from build123d import *

# Parameters (mm, degrees)
F1_DEPTH = 16
F2_T     = -1.5
F4_DEPTH = 100
F6_DEPTH = 25
F7_R     = 2


with BuildPart() as f1:
    # F0 (on Front) → F1 (new body)
    with BuildSketch(Plane.XZ):
        Polygon((32.5, -9), (32.5, 9), (-32.5, 9), (-32.5, -9), (-6, -9), (-6, -32), (6, -32), (6, -9), align=None)
    extrude(amount=F1_DEPTH)

    # F2
    f2_openings = [f1.faces().sort_by_distance(p)[0] for p in [
        (0, -16, -3.912863),
    ]]
    offset(amount=F2_T, openings=f2_openings, kind=Kind.INTERSECTION)

    # F3 (on face) → F4 (cut)
    with BuildSketch(Plane.YZ.offset(32.5)):
        with BuildLine():
            ThreePointArc((-7.5, -5), (-3.9644660941, -3.5355339059), (-2.5, 0))
            ThreePointArc((-2.5, 0), (-3.9336885694, 3.5044860935), (-7.4125691119, 4.9992355255))
            Line((-7.4125691119, 4.9992355255), (-7.5874308881, 4.9992355255))
            ThreePointArc((-7.5874308881, 4.9992355255), (-12.4994020552, 0.0773245797), (-7.7419960904, -4.9941403557))
            Line((-7.7419960904, -4.9941403557), (-7.5, -5))
        make_face()
        with BuildLine():
            Line((-7.5874308881, 4.9992355255), (-7.4125691119, 4.9992355255))
            ThreePointArc((-7.4125691119, 4.9992355255), (-7.5, 5), (-7.5874308881, 4.9992355255))
        make_face()
        with BuildLine():
            ThreePointArc((-7.7419960904, -4.9941403557), (-7.6210335111, -4.9985348743), (-7.5, -5))
            Line((-7.5, -5), (-7.7419960904, -4.9941403557))
        make_face()
        with BuildLine():
            ThreePointArc((-7.7419960904, -4.9941403557), (-12.4994020552, 0.0773245797), (-7.5874308881, 4.9992355255))
            Line((-7.5874308881, 4.9992355255), (-16, 4.9992355255))
            Line((-16, 4.9992355255), (-16, -4.7941827215))
            Line((-16, -4.7941827215), (-7.7419960904, -4.9941403557))
        make_face()
    extrude(amount=-F4_DEPTH, mode=Mode.SUBTRACT)

    # F5 (on face) → F6 (cut)
    with BuildSketch(Plane(origin=(0, 0, -32), x_dir=(1, 0, 0), z_dir=(0, 0, -1))):
        with BuildLine():
            ThreePointArc((-3.5, 6), (0, 2.5), (3.5, 6))
            ThreePointArc((3.5, 6), (0, 9.5), (-3.5, 6))
        make_face()
        with BuildLine():
            ThreePointArc((-3.5, 6), (0, 9.5), (3.5, 6))
            Line((3.5, 6), (3.5, 16))
            Line((3.5, 16), (-3.5, 16))
            Line((-3.5, 16), (-3.5, 6))
        make_face()
    extrude(amount=-F6_DEPTH, mode=Mode.SUBTRACT)

    # F7
    f7_edges = [f1.edges().sort_by_distance(p)[0] for p in [
        (-32.5, -8, -9),
        (-6, -8, -9),
        (-6, -8, -32),
        (6, -8, -32),
        (6, -8, -9),
        (32.5, -8, -9),
        (32.5, -8, 9),
        (-32.5, -8, 9),
    ]]
    fillet(f7_edges, radius=F7_R)


solid = f1.part
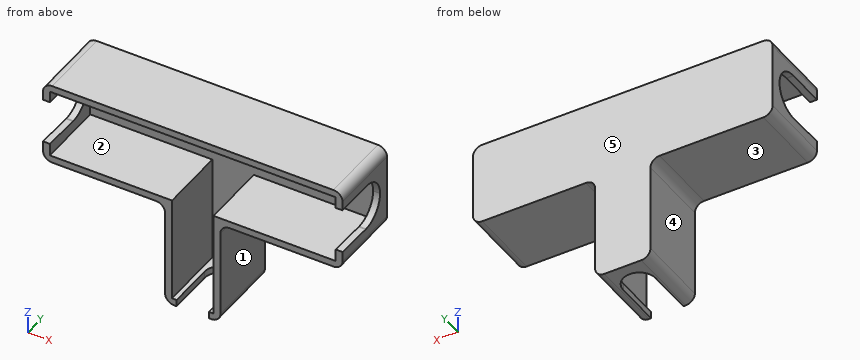
Read the model definition and answer for the solid it produces. Units are mm, in the model's axes. Face numbers are marked on the shaded views. A direction names the side the tool comes from. Round coordinates to 2 decimals unless told otherwise and drop trailing zeros. Order: outer loops, then holes, each group sorted by start corner. A loop starts at its lowest first (then second) coordinate and runs counter-clockwise, first axis right, second up.
1) Flat-ended cylindrical pins translate along their axes: pin 1 (7 mm diameter, centred on y = -6.5, z = -1.5, fed in from +X); pin 2 (1.2 mm diameter, centred on x = -32, y = -11.5, fed in from -Z); pin 3 (6 mm diameter, centred on x = -17, y = -7, fed in from -Z); pin 4 (8 mm diameter, centred on y = -8.5, z = -16.5, fed in from -X). Find the tip coordinate at first contact, or state that the pin passes through.
2) The mould has two halves that part along Y. Classify the marked faces 4 and 5: released by +Y, released by -Y, zero draft, split by the parting line, or undercut.
3) The part is cut by section A-A on x = -25.5. Write down the section's boundary in (y, z).
4) The part is cut by section B-B on z = -17.5. Write down the section's boundary in (x, y), plus the area to 3 significant figures.
5) Straight lines are drawn through the part: L1, parallel to Z at x = -16, y = -2.25; L2, parallel to X at y = -9.25, z = 7; L3, parallel to X at y = -4, z = -16.5. For each, find the intervals that lie inside material, in ascending order.
6) For the marked faces 1, 2 and 3, determine the directions among +Z, -Z, +X, -X, +Y, -Y from which every point of the face is accessible in a straight line to the end or side of a thin tool.
7) The part is cut by section C-C on y = -12.75. Give the number of separate pieces and of enclosed holes in the cut face, plus the area to 3 significant figures.
Resolved:
1. pin 1: stops at x = 32.5
1. pin 2: stops at z = -8.79
1. pin 3: stops at z = -9
1. pin 4: stops at x = -6
2. face 4: zero draft
2. face 5: released by +Y
3. outline: (-16, -9) - (0, -9) - (0, 9) - (-16, 9) - (-16, 7.5) - (-1.5, 7.5) - (-1.5, -7.5) - (-16, -7.5) - close
4. outline: (-6, -16) - (-4.5, -16) - (-4.5, -1.5) - (4.5, -1.5) - (4.5, -16) - (6, -16) - (6, 0) - (-6, 0) - close
4. area: 61.5 mm2
5. L1: z = -9 to -7.5, 7.5 to 9
5. L2: x = -32.5 to -31, 31 to 32.5
5. L3: x = -6 to -4.5, 4.5 to 6
6. face 1: -Z, +X, +Y, -Y
6. face 2: -Y
6. face 3: -Z, -X, +Y, -Y
7. separate pieces: 3
7. enclosed holes: 0
7. area: 265 mm2
